from build123d import *

# Parameters (mm, degrees)
CROQUIS2_W              = 16
CROQUIS2_H              = 2
SALIENTE_EXTRUIR3_DEPTH = 25
CROQUIS3_W              = 16
CROQUIS3_H              = 27
SALIENTE_EXTRUIR4_DEPTH = 2
REDONDEO1_R             = 2
CROQUIS4_R              = 3.25
CORTAR_EXTRUIR1_DEPTH   = 38.656340768
CROQUIS5_R              = 3.25
CORTAR_EXTRUIR2_DEPTH   = 37.945906404


with BuildPart() as part:
    # Croquis2 → Saliente-Extruir3 (new body)
    with BuildSketch(Plane(origin=(0, 0, 0), x_dir=(0, 0, -1), z_dir=(1, 0, 0))):
        Rectangle(CROQUIS2_W, CROQUIS2_H)
    extrude(amount=SALIENTE_EXTRUIR3_DEPTH)

    # Croquis3 → Saliente-Extruir4 (add)
    with BuildSketch(Plane(origin=(25, 0, 0), x_dir=(0, 0, -1), z_dir=(1, 0, 0))):
        with Locations((0, 12.5)):
            Rectangle(CROQUIS3_W, CROQUIS3_H)
    extrude(amount=SALIENTE_EXTRUIR4_DEPTH)

    # Redondeo1
    redondeo1_edges = [part.edges().sort_by_distance(p)[0] for p in [
        (27, -1, 0),
        (25, 1, 0),
    ]]
    fillet(redondeo1_edges, radius=REDONDEO1_R)

    # Croquis4 → Cortar-Extruir1 (cut, through all)
    with BuildSketch(Plane(origin=(0, 1, 0), x_dir=(1, 0, 0), z_dir=(0, 1, 0))):
        with Locations(Location((9.25, 0, 0), (0, 0, 270))):
            Circle(CROQUIS4_R)
    extrude(amount=-CORTAR_EXTRUIR1_DEPTH, mode=Mode.SUBTRACT)

    # Croquis5 → Cortar-Extruir2 (cut, through all)
    with BuildSketch(Plane.ZY.offset(-25)):
        with Locations((0, 20)):
            Circle(CROQUIS5_R)
    extrude(amount=-CORTAR_EXTRUIR2_DEPTH, mode=Mode.SUBTRACT)


solid = part.part
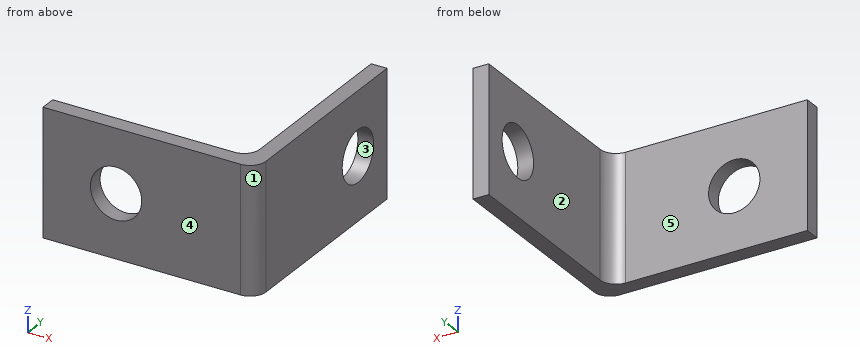
Build history of the part. All positions in model axes, mm. Face numbers are marked on the shaded views. A direction names the side the tool comes from. Give positions to 0.01 mm unless a question says otherwise; leave off trailing zeros. Loops run counter-clockwise (first coordinate to the right, second up) from the corner with the lowest first, then second, coordinate; pieces in that order, holes last. Notation, with made-up numbers: (40.25, -27) -> (98.25, -27) arc R30 ccw to (98.25, 2) -> close; hole circle Ø10 at (-31, -31.75). An arc over 180 degrees is marked (long way). Answer in a Markdown table with one row per item.
Item 1: Tool access for the marked faces 4 and 5: list every direction of +Z, -Z, +X, -X, +Y, -Y with a clear straight run to the whole face (end or side of a thin tool).
Findings below:
| item | result |
|---|---|
| face 4 | +Z, -Z, +X, -X, -Y |
| face 5 | +Z, -Z, -X, +Y |
Item 2: Slice it at D-D on z = 6. Write the cut outline in (x, y).
Findings below:
| item | result |
|---|---|
| outline | (0, -1) -> (25, -1) arc R2 ccw to (27, 1) -> (27, 26) -> (25, 26) -> (25, 3) arc R2 cw to (23, 1) -> (0, 1) -> close |
Item 3: Slice it at C-C on z = 0. Write the cut outline in (x, y), plus the area to 3 significant figures.
Findings below:
| item | result |
|---|---|
| outline | (0, -1) -> (6, -1) -> (6, 1) -> (0, 1) -> close; (12.5, -1) -> (25, -1) arc R2 ccw to (27, 1) -> (27, 16.75) -> (25, 16.75) -> (25, 3) arc R2 cw to (23, 1) -> (12.5, 1) -> close; (25, 23.25) -> (27, 23.25) -> (27, 26) -> (25, 26) -> close |
| area | 78.0 mm² |
Item 4: Flat gauge pins, fed straight in: P1, Ø8, axis at x = 14, z = 0, coming from the +Y side; P2, Ø5, axis at y = 20, z = 0, coming from the -X side; P3, Ø6, axis at y = 6.5, z = 3, coming from the -X side. Where does each tip first touch, or does it go through?
Findings below:
| item | result |
|---|---|
| P1 | stops at y = 1 |
| P2 | passes through |
| P3 | stops at x = 25 |
Item 5: Probe line 1 along Y through (x, z) = (14.25, -4.25); line 2 along X through (y, z) = (14.5, -3); line 3 along X through (y, z) = (0.4, 0). List the from-to ranges inside material, lowest first. Write a range as [from, to].
Findings below:
| item | result |
|---|---|
| line 1 | y = [-1, 1] |
| line 2 | x = [25, 27] |
| line 3 | x = [0, 6], [12.5, 26.91] |
Item 6: Slice it at B-B on x = 9.25. Write the cut outline in (y, z), plus the area to 3 significant figures.
Findings below:
| item | result |
|---|---|
| outline | (-1, -8) -> (1, -8) -> (1, -3.25) -> (-1, -3.25) -> close; (-1, 3.25) -> (1, 3.25) -> (1, 8) -> (-1, 8) -> close |
| area | 19.0 mm² |
Item 7: Slice it at A-A on y = 20. Write the cut outline in (x, z).
Findings below:
| item | result |
|---|---|
| outline | (25, -8) -> (27, -8) -> (27, -3.25) -> (25, -3.25) -> close; (25, 3.25) -> (27, 3.25) -> (27, 8) -> (25, 8) -> close |
Item 8: Mould opens along Y. For the marked faces 1, 2 and 3 say: pulls with the +Y half, pulls with the -Y half, needs draft (parallel to the pull), parting line crosses it, or undercut.
Findings below:
| item | result |
|---|---|
| face 1 | pulls with the -Y half |
| face 2 | needs draft |
| face 3 | undercut |
